from build123d import *

# Parameters (mm, degrees)
F0_W      = 69.85
F0_H      = 100.5
F1_DEPTH  = 7
F2_R      = 3
F3_R      = 1.5
F4_DEPTH  = 5
F5_R      = 1.5
F6_DEPTH  = 5
F7_W      = 40
F7_H      = 10
F8_DEPTH  = 3
F9_R      = 1.5
F10_DEPTH = 5


with BuildPart() as f1:
    # F0 (on Top) → F1 (new body)
    with BuildSketch(Plane.XY):
        Rectangle(F0_W, F0_H)
    extrude(amount=F1_DEPTH)

    # F2
    f2_edges = [f1.edges().sort_by_distance(p)[0] for p in [
        (34.925, 50.25, 3.5),
        (-34.925, 50.25, 3.5),
        (34.925, -50.25, 3.5),
        (-34.925, -50.25, 3.5),
    ]]
    fillet(f2_edges, radius=F2_R)

    # F3 (on face) → F4 (cut)
    with BuildSketch(Plane.YZ.offset(34.925)):
        with Locations((-36.25, 3)):
            Circle(F3_R)
        with Locations((40.35, 3)):
            Circle(F3_R)
    extrude(amount=-F4_DEPTH, mode=Mode.SUBTRACT)

    # F5 (on face) → F6 (cut)
    with BuildSketch(Plane(origin=(-34.925, 0, 0), x_dir=(0, -1, 0), z_dir=(-1, 0, 0))):
        with Locations((36.25, 3)):
            Circle(F5_R)
        with Locations((-40.35, 3)):
            Circle(F5_R)
    extrude(amount=-F6_DEPTH, mode=Mode.SUBTRACT)

    # F7 (on face) → F8 (cut)
    with BuildSketch(Plane(origin=(0, 0, 0), x_dir=(1, 0, 0), z_dir=(0, 0, -1))):
        with Locations((0, 45.25)):
            Rectangle(F7_W, F7_H)
    extrude(amount=-F8_DEPTH, mode=Mode.SUBTRACT)

    # F9 (on face) → F10 (cut)
    with BuildSketch(Plane(origin=(0, 0, 0), x_dir=(1, 0, 0), z_dir=(0, 0, -1))):
        with Locations((-30.855, 36.25)):
            Circle(F9_R)
        with Locations((-30.855, -40.35)):
            Circle(F9_R)
        with Locations((30.855, -40.35)):
            Circle(F9_R)
        with Locations((30.855, 36.25)):
            Circle(F9_R)
    extrude(amount=-F10_DEPTH, mode=Mode.SUBTRACT)


solid = f1.part
Work out the finished part from the listing and answer in its coordinate system (mm). A direction names the side the tool comes from. Coordinates: 2 decimals unless noted, no trailing zeros. Write each loop counter-clockwise with the first axis right and the second up, starting at its lowest first coordinate (ties: lowest second). Pieces come first, ordered by that corner, then holes. Notation, with made-up numbers: M 3,49.25 L 16,49.25 A28 cw 16,80.25 Z; hole C 61.5,-38 d5. An arc over 180 degrees is marked long. Answer as CSV lines item,"result". Start each with the question number.
Item 1: A tool of negligible diameter and unlimited length cuts with its end or side. For faces 1 (the face through (-33.37, -34.75, 3.07)), 2 (the face through (29.356, 40.284, 2.465)), 3 (the face through (20, -45, 1)), 4 (the face through (33.37, -37.75, 3.07)), from which of +Z, -Z, +X, -X, +Y, -Y can it reach the whole face along a straight path? Write none if from no direction.
Item 2: Consider L1, parallel to Y at x = -30.5, z = 3; L2, parallel to Z at x = 32.6, y = -36.25; L3, parallel to Y at x = -29.5, z = 3.75. Determine where each line is inside the solid, lowest interval first.
Item 3: Section A-A on y = -36.25 is taken. Write down the section's boundary in (x, z) (3 decimals).
Item 4: Flat-ended cylindrical pins translate along their axes: P1, Ø3.5, axis at x = -31.5, y = -36.5, coming from the -Z side; P2, Ø1.5, axis at x = 8.5, z = 1.5, coming from the -Y side; P3, Ø2.5, axis at y = -36.25, z = 3, coming from the +X side (3 decimals); P4, Ø2.5, axis at y = 40.35, z = 3, coming from the -X side (3 decimals). Find the tip coordinate at first contact, or state that the pin passes through.
Item 5: Section B-B on x = -14 is taken. Write down the section's boundary in (y, z).
Item 6: Determine the mould class of faces 5 (the face through (-34.07, -49.35, 3.55)), 6 (the face through (-31, 40, 5)), 7 (the face through (0, 1, 7)) for opening direction Y: released by +Y, released by -Y, zero draft, split by the parting line, or undercut.
Checks:
1,face 1,"-X"
1,face 2,"-Z"
1,face 3,"-Z, -Y"
1,face 4,"+X"
2,L1,"y = -50.25 to -37.75, -34.75 to 38.85, 41.85 to 50.25"
2,L2,"z = 0 to 1.5, 4.5 to 7"
2,L3,"y = -50.25 to -36.89, -35.61 to 39.71, 40.99 to 50.25"
3,outline,"M -34.925,0 L -32.355,0 L -32.355,1.5 L -34.925,1.5 Z; M -34.925,4.5 L -32.355,4.5 L -32.355,5 L -29.355,5 L -29.355,0 L 29.355,0 L 29.355,5 L 32.355,5 L 32.355,4.5 L 34.925,4.5 L 34.925,7 L -34.925,7 Z; M 32.355,0 L 34.925,0 L 34.925,1.5 L 32.355,1.5 Z"
4,P1,"stops at z = 0"
4,P2,"stops at y = -40.25"
4,P3,"stops at x = 29.925"
4,P4,"stops at x = -29.925"
5,outline,"M -50.25,3 L -40.25,3 L -40.25,0 L 50.25,0 L 50.25,7 L -50.25,7 Z"
6,face 5,"released by -Y"
6,face 6,"undercut"
6,face 7,"zero draft"
